Model file for the job. Use its own axes, mm. Face numbers are marked on the shaded views. A direction names the side the tool comes from. Give positions to 0.01 mm unless a question says otherwise; leave off trailing zeros. Order: outer loops, then holes, each group sorted by start corner. A loop starts at its lowest first (then second) coordinate and runs counter-clockwise, first axis right, second up. Notation, with made-up numbers: (15, 50) -> (69, 50) arc R8 ccw to (69, 63) -> close; hole circle Ø2 at (-17.75, 0). An arc over 180 degrees is marked (long way). Use CSV: the item, a comma, the result in double quotes. Start each with the question number.
1. Pull direction Y, two halves, no side cores. Call the marked faces 3, 4 and 5: released by +Y, released by -Y, zero draft, split by the parting line, or undercut.
2. Drop flat-ended pins along their axis: pin 1 (5 mm diameter, centred on x = -3.5, y = 14, fed in from -Z); pin 2 (6 mm diameter, centred on y = -13.5, z = 24, fed in from -X); pin 3 (4 mm diameter, centred on x = -7, y = -5, fed in from -Z). Give the stop position or say it passes through.
3. Cut at A-A on y = 0. List the corners of the cut face in (x, z) (3 decimals), then the cut area to 3 significant figures.
4. 3-axis set-ups, long thin cutter, end or side, ignore diameter. For the marked faces 1 and 2: which of +Z, -Z, +X, -X, +Y, -Y reach the whole face in a straight line?
5. Cut at C-C on z = 9. List the corners of the cut face in (x, y), then the cut area to 3 significant figures.
6. Cut at B-B on x = -5.75. Give the number of separate pieces and of enclosed holes in the cut face, then the cut area to 3 significant figures.
7. Wall check: line 1 (Z direction, x = -2.25, y = 13); line 2 (Y direction, x = -2, z = 20); line 3 (Z direction, x = -4.5, y = 16). Give the ranges that are in metal, low to high. Write a range as from..to.
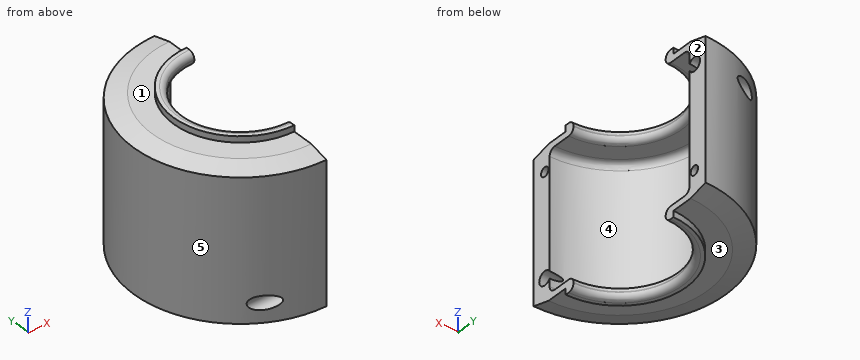
```python
from build123d import *

# Parameters (mm, degrees)
F1_ANGLE = 180
F3_DEPTH = 27.813
F4_R     = 1.016
F5_R     = 1.0922
F7_D     = 2.3622
F8_D     = 1.5748
F8_DEPTH = 6.35
F8_TIP   = 0.4731176514
F9_SIZE2 = 3.175
F9_SIZE  = 0.850738686


with BuildPart() as f1:
    # F0 (on Right) → F1 (revolve)
    with BuildSketch(Plane.YZ):
        Polygon((0, 2.1336), (0, 0), (11.43, 0), (11.43, 1.0414), (18.2372, 1.0414), (18.2372, 26.7716), (11.43, 26.7716), (11.43, 27.813), (0, 27.813), (0, 25.6794), (14.859, 25.6794), (14.859, 2.1336), align=None)
    revolve(axis=Axis((0, 0, 26.7462), (0, 0, 1)), revolution_arc=F1_ANGLE)

    # F2 (on face) → F3 (cut)
    with BuildSketch(Plane.XY.offset(27.813)):
        with BuildLine():
            ThreePointArc((0, -9.779), (6.9147972132, -6.9147972132), (9.779, 0))
            ThreePointArc((9.779, 0), (6.9147972132, 6.9147972132), (0, 9.779))
            Line((0, 9.779), (0, -9.779))
        make_face()
        with BuildLine():
            Line((0, -9.779), (0, 9.779))
            ThreePointArc((0, 9.779), (-9.779, 0), (0, -9.779))
        make_face()
    extrude(amount=-F3_DEPTH, mode=Mode.SUBTRACT)

    # F4
    f4_edges = [f1.edges().sort_by_distance(p)[0] for p in [
        (-9.779, 0, 27.813),
        (-9.779, 0, 25.6794),
        (-9.779, 0, 2.1336),
        (-9.779, 0, 0),
    ]]
    fillet(f4_edges, radius=F4_R)

    # F5
    f5_edges = [f1.edges().sort_by_distance(p)[0] for p in [
        (-14.859, 0, 25.6794),
        (-14.859, 0, 2.1336),
    ]]
    fillet(f5_edges, radius=F5_R)

    # F7 (through all)
    with Locations(Plane.YZ):
        with Locations((15.875, 22.6314), (-15.875, 5.1816)):
            Hole(F7_D / 2)

    # F8
    with Locations(Plane.YZ):
        with Locations((15.875, 5.1816), (-15.875, 22.6314)):
            Hole(F8_D / 2, depth=F8_DEPTH)
            with Locations((0, 0, -(F8_DEPTH + F8_TIP / 2))):  # 118° drill point
                Cone(0, F8_D / 2, F8_TIP, mode=Mode.SUBTRACT)

    # F9
    f9_edges = [f1.edges().sort_by_distance(p)[0] for p in [
        (-18.2372, 0, 1.0414),
        (-18.2372, 0, 26.7716),
    ]]
    f9_side = f1.faces().sort_by_distance((-18.2372, 0, 13.9065))[0]
    chamfer(f9_edges, length=F9_SIZE, length2=F9_SIZE2, reference=f9_side)


solid = f1.part
```
Verdict:
1,face 3,"zero draft"
1,face 4,"undercut"
1,face 5,"split by the parting line"
2,pin 1,"z = 1.04"
2,pin 2,"x = -14.91"
2,pin 3,"z = 0.02"
3,outline,"(-18.237, 1.892) -> (-15.062, 1.041) -> (-11.43, 1.041) -> (-11.43, 0) -> (-10.795, 0) arc R1.016 ccw to (-9.779, 1.016) -> (-9.779, 1.118) arc R1.016 ccw to (-10.795, 2.134) -> (-13.767, 2.134) arc R1.092 cw to (-14.859, 3.226) -> (-14.859, 24.587) arc R1.092 cw to (-13.767, 25.679) -> (-10.795, 25.679) arc R1.016 ccw to (-9.779, 26.695) -> (-9.779, 26.797) arc R1.016 ccw to (-10.795, 27.813) -> (-11.43, 27.813) -> (-11.43, 26.772) -> (-15.062, 26.772) -> (-18.237, 25.921) -> close"
3,area,"98.4 mm^2"
4,face 1,"+Z, -X"
4,face 2,"+Z, -Z, +X, +Y, -Y"
5,outline,"(0, -18.24) -> (0, -14.86) arc R14.86 cw to (0, 14.86) -> (0, 18.24) arc R18.24 ccw to start"
5,area,"176 mm^2"
6,separate pieces,"2"
6,enclosed holes,"4"
6,area,"200 mm^2"
7,line 1,"1.04..2.13, 25.68..26.77"
7,line 2,"-18.13..-14.72, 14.72..18.13"
7,line 3,"1.46..4.4, 5.96..21.46, 23.81..26.35"
